Design review of the part built by this model. Coordinates are the model's own, in mm. Give positions to 0.01 mm unless a question says otherwise; leave off trailing zeros. Order: outer loops, then holes, each group sorted by start corner. A loop starts at its lowest first (then second) coordinate and runs counter-clockwise, first axis right, second up. Notation, with made-up numbers: (-33.75, 1.25) -> (18.25, 1.25) arc R12 cw to (18.25, 15.25) -> close; hole circle Ø1 at (17, 29.5). An arc over 180 degrees is marked (long way). Return JSON: item names as keys, results as strings.
```python
from build123d import *

# Parameters (mm, degrees)
SKETCH4_W                = 68.600000001
SKETCH4_H                = 53.4
BRACKETBASE_DEPTH        = 5
MOUNTINGHOLES_DEPTH      = 79.489210088
MOUNTINGHOLES_DEPTH_BACK = 79.489210088
MOUNTINGHOLESSKETCH_R    = 1.25


with BuildPart() as part:
    # Sketch4 → bracketBase (new body)
    with BuildSketch(Plane.XY):
        with Locations((34.3, 11.110000001)):
            Rectangle(SKETCH4_W, SKETCH4_H)
    extrude(amount=BRACKETBASE_DEPTH)

    # mountingHolesSketch → mountingHoles (cut, two sides: drawn at the far end of the back side and taken through both)
    with BuildSketch(Plane.XY.offset(-MOUNTINGHOLES_DEPTH_BACK)):
        with Locations((2.54, 2.280000001)):
            Circle(MOUNTINGHOLESSKETCH_R)
        with Locations((2.54, 30.450000001)):
            Circle(MOUNTINGHOLESSKETCH_R)
        with Locations((54.600000001, 35.270000001)):
            Circle(MOUNTINGHOLESSKETCH_R)
        with Locations((53.350000001, -13.049999999)):
            Circle(MOUNTINGHOLESSKETCH_R)
    extrude(amount=MOUNTINGHOLES_DEPTH + MOUNTINGHOLES_DEPTH_BACK, mode=Mode.SUBTRACT)


solid = part.part
```
Item 1: Mouldability with a two-part tool opening along X and no side actions: class faces 1 (the face through (0, 11, 2)), 2 (the face through (2.27, 29.23, 2.47)), 3 (the face through (34, 11, 0)) as released by +X, released by -X, zero draft, split by the parting line, or undercut.
Result set:
{"face 1": "released by -X", "face 2": "undercut", "face 3": "zero draft"}
Item 2: Wall thickness on L1, parallel to Y at x = 2.54, z = 1.3; L2, parallel to X at y = 2, z = 0.25: over which ranges is each line inside the solid? List them lowest first. Write a range as [from, to].
Result set:
{"L1": "y = [-15.59, 1.03], [3.53, 29.2], [31.7, 37.81]", "L2": "x = [0, 1.32], [3.76, 68.6]"}
Item 3: Add section B-B (y = 30.45). Give the boundary of the cut face in (x, z), plus the area to 4 significant figures.
Result set:
{"outline": "(0, 0) -> (1.29, 0) -> (1.29, 5) -> (0, 5) -> close; (3.79, 0) -> (68.6, 0) -> (68.6, 5) -> (3.79, 5) -> close", "area": "330.5 mm^2"}
Item 4: Add section A-A (x = 2.54). Give the boundary of the cut face in (y, z), plus the area to 3 significant figures.
Result set:
{"outline": "(-15.59, 0) -> (1.03, 0) -> (1.03, 5) -> (-15.59, 5) -> close; (3.53, 0) -> (29.2, 0) -> (29.2, 5) -> (3.53, 5) -> close; (31.7, 0) -> (37.81, 0) -> (37.81, 5) -> (31.7, 5) -> close", "area": "242 mm^2"}
